Design review of the part built by this model. Coordinates are the model's own, in mm. A direction names the side the tool comes from. Give positions to 0.01 mm unless a question says otherwise; leave off trailing zeros. Order: outer loops, then holes, each group sorted by start corner. A loop starts at its lowest first (then second) coordinate and runs counter-clockwise, first axis right, second up. Notation, with made-up numbers: M 64.25,71.5 L 84.25,71.5 A17 cw 84.25,99.5 Z; hole C 29.5,52.5 d11. An arc over 180 degrees is marked long. Put each result on its own line as item: value. Start each with the question number.
from build123d import *

# Parameters (mm, degrees)
CHAMFER_1_SIZE = 0.2
M3X0_5_2_D     = 2.5
M3X0_5_2_DEPTH = 4
M3X0_5_2_TIP   = 0.751075774
M3X0_5_3_D     = 2.5
M3X0_5_3_DEPTH = 4
M3X0_5_3_TIP   = 0.751075774
M3X0_5_4_D     = 2.5


with BuildPart() as part:
    # 草图2 → 旋转1 (revolve)
    with BuildSketch(Plane(origin=(0, 0, 0), x_dir=(1, 0, 0), z_dir=(0, 1, 0))):
        Polygon((-77.680952315, 55.25), (-72.180952315, 55.25), (-72.180952315, 49.25), (-69.180952315, 49.25), (-69.180952315, 47.85), (-63.680952315, 47.85), (-63.680952315, 49.25), (-59.680952315, 49.25), (-59.680952315, 47.85), (-54.180952315, 47.85), (-54.180952315, 49.25), (-49.180952315, 49.25), (-49.180952315, 42.25), (-77.680952315, 42.25), (-77.680952315, 46.2), (-76.780952315, 46.2), (-76.780952315, 49.8), (-77.680952315, 49.8), align=None)
    revolve(axis=Axis((0, 0, 0), (-1, 0, 0)))

    # 倒角1
    chamfer_1_edges = [part.edges().sort_by_distance(p)[0] for p in [
        (-77.680952315, 0, 49.8),
        (-77.680952315, 0, 46.2),
        (-54.180952315, 0, 49.25),
        (-59.680952315, 0, 49.25),
        (-63.680952315, 0, 49.25),
        (-69.180952315, 0, 49.25),
    ]]
    chamfer(chamfer_1_edges, length=CHAMFER_1_SIZE)

    # M3x0.5 螺纹孔2
    with Locations(Plane(origin=(-49.180952315, 45.75, 0), x_dir=(0, 0, 1), z_dir=(1, 0, 0))):
        with Locations((0, 0)):
            Hole(M3X0_5_2_D / 2, depth=M3X0_5_2_DEPTH)
            with Locations((0, 0, -(M3X0_5_2_DEPTH + M3X0_5_2_TIP / 2))):  # 118° drill point
                Cone(0, M3X0_5_2_D / 2, M3X0_5_2_TIP, mode=Mode.SUBTRACT)

    # M3x0.5 螺纹孔3
    with Locations(Plane(origin=(-49.180952315, 0, -45.75), x_dir=(0, 0, 1), z_dir=(1, 0, 0))):
        with Locations((0, 0), (91.5, 0), (45.75, 45.75)):
            Hole(M3X0_5_3_D / 2, depth=M3X0_5_3_DEPTH)
            with Locations((0, 0, -(M3X0_5_3_DEPTH + M3X0_5_3_TIP / 2))):  # 118° drill point
                Cone(0, M3X0_5_3_D / 2, M3X0_5_3_TIP, mode=Mode.SUBTRACT)

    # M3x0.5 螺纹孔4 (through all)
    with Locations(Plane(origin=(-77.680952315, 52.525, 0), x_dir=(0, 0, -1), z_dir=(-1, 0, 0))):
        with Locations((0, 0), (-45.487984334, 26.2625), (-45.487984334, 78.7875), (0, 105.05), (45.487984334, 78.7875), (45.487984334, 26.2625)):
            Hole(M3X0_5_4_D / 2)


solid = part.part
1. To check wall thickness, follow probe 1 along Y at (x, z) = (-51.35, 0); probe 2 along Y at (x, z) = (-77.05, 0) (3 decimals); probe 3 along Y at (x, z) = (-75.65, 0) (3 decimals). State the ranges of each line that lie inside material, in increasing order.
2. Insertion check: pin 1 (5 mm diameter, centred on x = -69, z = -40.5, fed in from +Y); pin 2 (4 mm diameter, centred on y = 0, z = -45.75, fed in from +X); pin 3 (8 mm diameter, centred on x = -55, z = 12, fed in from -Y); pin 4 (2 mm diameter, centred on x = -55.5, z = 15.5, fed in from -Y). Each pin has a flat end and moves straight along its axis. Give the tip position at first contact, or say it passes through.
3. Consider section A-A on x = -56. Give the boundary of the cut face in (y, z), then the cut area to 3 significant figures.
4. Machinability: for faces 5 (the flat face through (-76.781, 15, 44)), 6 (the cylindrical face through (-51, -47, 0)), 7 (the flat face through (-63.681, 47, 11)), which of the approach directions +Z, -Z, +X, -X, +Y, -Y give a long, thin tool a straight path to every point of the face, cutting with its end or side? Answer none if there is none.
5. The part is to be moulded in two halves that separate along X. For faces 1 (the flat face through (-49.181, -37, -22)), 2 (the flat face through (-77.681, -41, -29)), 3 (the flat face through (-54.181, 47, 11)), 4 (the cylindrical face through (-51.21, -0.05, -44.5)), say which applies: +X half, -X half, draft (parallel to the pull), parting line (faces both ways), or undercut.
Returned:
1. probe 1: y = -49.25 to -47, -44.5 to -42.25, 42.25 to 44.5, 47 to 49.25
1. probe 2: y = -55.25 to -53.775, -51.275 to -49.8, -46.2 to -42.25, 42.25 to 46.2, 49.8 to 51.275, 53.775 to 55.25
1. probe 3: y = -55.25 to -53.775, -51.275 to -42.25, 42.25 to 51.275, 53.775 to 55.25
2. pin 1: stops at y = 31.29
2. pin 2: stops at x = -49.18
2. pin 3: stops at y = -48.57
2. pin 4: stops at y = -45.6
3. outline: C 0,0 d95.7; hole C 0,0 d84.5
3. area: 1,590 mm2
4. face 5: -X
4. face 6: +X
4. face 7: none
5. face 1: +X half
5. face 2: -X half
5. face 3: undercut
5. face 4: draft
